from build123d import *

# Parameters (mm, degrees)
ESQUISSE1_W             = 55
ESQUISSE1_H             = 150
BOSS_EXTRU_1_DEPTH      = 20
ESQUISSE2_W             = 50
ESQUISSE2_H             = 10
ENL_V_MAT_EXTRU_1_DEPTH = 162.012421881
ESQUISSE3_R             = 4
ENL_V_MAT_EXTRU_2_DEPTH = 20
CONG_1_R                = 5
CONG_2_R                = 10
CONG_3_R                = 10


with BuildPart() as part:
    # Esquisse1 → Boss.-Extru.1 (new body)
    with BuildSketch(Plane.XY):
        with Locations((-27.5, 75)):
            Rectangle(ESQUISSE1_W, ESQUISSE1_H)
    extrude(amount=BOSS_EXTRU_1_DEPTH)

    # Esquisse2 → Enlèv. mat.-Extru.1 (cut, through all)
    with BuildSketch(Plane(origin=(0, 150, 0), x_dir=(1, 0, 0), z_dir=(0, 1, 0))):
        with Locations((-30, -10)):
            Rectangle(ESQUISSE2_W, ESQUISSE2_H)
    extrude(amount=-ENL_V_MAT_EXTRU_1_DEPTH, mode=Mode.SUBTRACT)

    # Esquisse3 → Enlèv. mat.-Extru.2 (cut)
    with BuildSketch(Plane(origin=(0, 0, 0), x_dir=(-1, 0, 0), z_dir=(0, 0, -1))):
        with Locations((27.5, 136.25286599)):
            Circle(ESQUISSE3_R)
    extrude(amount=-ENL_V_MAT_EXTRU_2_DEPTH, mode=Mode.SUBTRACT)

    # Congé1
    cong_1_edges = [part.edges().sort_by_distance(p)[0] for p in [
        (-5, 75, 15),
        (-5, 75, 5),
    ]]
    fillet(cong_1_edges, radius=CONG_1_R - 0.0001)  # a hair under: the kernel refuses the full size

    # Congé2
    cong_2_edges = [part.edges().sort_by_distance(p)[0] for p in [
        (0, 75, 0),
        (0, 75, 20),
    ]]
    fillet(cong_2_edges, radius=CONG_2_R - 0.0001)  # a hair under: the kernel refuses the full size

    # Congé3
    cong_3_edges = [part.edges().sort_by_distance(p)[0] for p in [
        (-55, 0, 2.5),
        (-55, 150, 2.5),
        (-55, 0, 17.5),
        (-55, 150, 17.5),
    ]]
    fillet(cong_3_edges, radius=CONG_3_R)


solid = part.part
Build history of the part. All positions in model axes, mm. A direction names the side the tool comes from. Coordinates: 2 decimals unless noted, no trailing zeros. Order: outer loops, then holes, each group sorted by start corner. A loop starts at its lowest first (then second) coordinate and runs counter-clockwise, first axis right, second up. Notation, with made-up numbers: (79, 74) - (137, 74) arc R17 cw to (137, 93) - close; hole circle Ø5 at (-10.75, 72). An arc over 180 degrees is marked (long way). Write each question's results on one line, items separated by ' | '. Start each with the question number.
Item 1: Band-saw the part on A-A on x = -27.5. Write the cut outline in (y, z).
Item 2: Flat gauge pin, fed straight in: pin 1 (1 mm diameter, centred on x = -34.5, z = 14, fed in from -Y). Where does the tip first touch, or does it go through?
Item 3: Band-saw the part on D-D on z = 2. Write the cut outline in (x, y).
Item 4: Tool access for faces 1 (the face through (-7, 74, 6)), 2 (the face through (-52.15, 3.01, 2.54)): list every direction of +Z, -Z, +X, -X, +Y, -Y with a clear straight run to the whole face (end or side of a thin tool).
Item 5: Wall check: probe 1 along Y at (x, z) = (-28, 16); probe 2 along Z at (x, y) = (-39, 86.5); probe 3 along X at (y, z) = (68, 17). Give the ranges that are in metal, low to high. Write a range as [from, to].
Item 6: Band-saw the part on B-B on x = -37. Write the cut outline in (y, z).
Item 7: Mould opens along Y. For faces 3 (the face through (-23, 0, 3)), 4 (the face through (-26.98, 140.22, 2.46)), 5 (the face through (-33, 76, 0)) say: released by +Y, released by -Y, zero draft, split by the parting line, or undercut.
Numbers:
1) outline: (0, 0) - (132.25, 0) - (132.25, 5) - (0, 5) - close; (0, 15) - (132.25, 15) - (132.25, 20) - (0, 20) - close; (140.25, 0) - (150, 0) - (150, 5) - (140.25, 5) - close; (140.25, 15) - (150, 15) - (150, 20) - (140.25, 20) - close
2) pin 1: through
3) outline: (-55, 10) arc R10 ccw to (-45, 0) - (-4, 0) - (-4, 150) - (-45, 150) arc R10 ccw to (-55, 140) - close; hole circle Ø8 at (-27.5, 136.25)
4) face 1: -X, +Y, -Y | face 2: +Z, -Z, -X, -Y
5) probe 1: [0, 132.28], [140.22, 150] | probe 2: [0, 5], [15, 20] | probe 3: [-55, -2.86]
6) outline: (0, 0) - (150, 0) - (150, 5) - (0, 5) - close; (0, 15) - (150, 15) - (150, 20) - (0, 20) - close
7) face 3: released by -Y | face 4: undercut | face 5: zero draft
